Autodesk Inventor part; units mm, degrees
ref_plane "YZ Plane" through (0, 0, 0) normal (1, 0, 0) x (0, 1, 0)
ref_plane "XZ Plane" through (0, 0, 0) normal (0, 1, 0) x (-1, 0, 0)
ref_plane "XY Plane" through (0, 0, 0) normal (0, 0, 1) x (1, 0, 0)
sketch "Sketch1" plane through (0, 0, 0) normal (0, 1, 0) x (-1, 0, 0)
  line L0 (-50.8, 50.8) -> (-50.8, -50.8)
  line L1 (-50.8, -50.8) -> (50.8, -50.8)
  line L2 (50.8, -50.8) -> (50.8, 50.8)
  line L3 (50.8, 50.8) -> (-50.8, 50.8)
  line L4 (-50.8, 50.8) -> (50.8, -50.8) construction
  line L5 (-50.8, -50.8) -> (50.8, 50.8) construction
  line L6 (-47.625, 47.625) -> (-47.625, -47.625)
  line L7 (-47.625, -47.625) -> (47.625, -47.625)
  line L8 (47.625, -47.625) -> (47.625, 47.625)
  line L9 (47.625, 47.625) -> (-47.625, 47.625)
  line L10 (-47.625, 47.625) -> (47.625, -47.625) construction
  line L11 (-47.625, -47.625) -> (47.625, 47.625) construction
  point P0 (0, 0)
  dimension "d0" = 101.6
  dimension "d1" = 3.175
extrude "Extrusion1" add sketch "Sketch1" along normal blind 609.6
properties part number "AlumPost-4x4x36-1_8" material "Aluminum 6061"
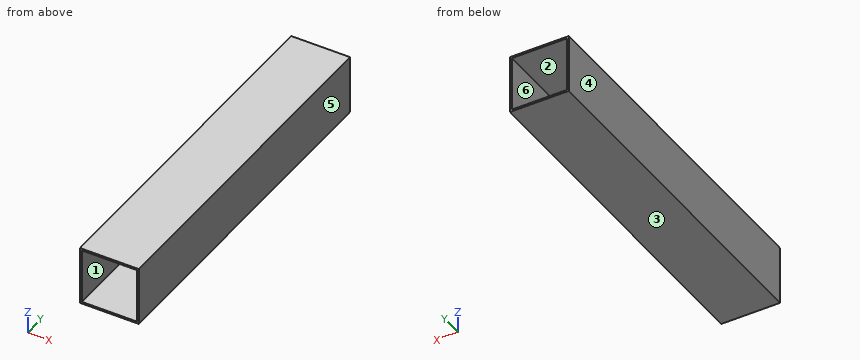
Can you work these out from the model? Positions are in its coordinate system, mm. Face numbers are marked on the shaded views. A direction names the side the tool comes from. Give positions to 0.01 mm unless a question says otherwise; leave off trailing zeros. Order: outer loops, then holes, each group sorted by start corner. A loop starts at its lowest first (then second) coordinate and runs counter-clockwise, first axis right, second up. Notation, with made-up numbers: M 57,25.25 L 79,25.25 A27 cw 79,52.25 Z; hole C 73,84 d9. An arc over 180 degrees is marked long. Use one line per item in the form item = value. Start each with the question number.
Item 1: If we section it at B-B (y = 546): Write out the boundary of the cut face in (x, z) (3 decimals).
Item 2: If we section it at C-C (x = -10): Write out the boundary of the cut face in (y, z) (3 decimals), then the cut area to 3 significant figures.
Item 3: If we section it at A-A (z = 11.5): Write out the boundary of the cut face in (x, y) (3 decimals).
Item 4: If I drill on line 1 along Z through (x, y) = (14.5, 42.5) (3 decimals), over which ranges is the centre line in solid material (lowest first)?
Item 5: For the marked faces 5 and 6, which set-ups out of +Z, -Z, +X, -X, +Y, -Y let a thin tool reach every point of the face, with its end or its side?
Item 6: We'd pull the mould along Z, two halves only. Please class the marked faces 1, 2, 3 and 4: +Z half, -Z half, draft (parallel to the pull), parting line (faces both ways), or undercut.
Outcome:
q1.outline = M -50.8,-50.8 L 50.8,-50.8 L 50.8,50.8 L -50.8,50.8 Z; hole M -47.625,-47.625 L 47.625,-47.625 L 47.625,47.625 L -47.625,47.625 Z
q2.outline = M 0,-50.8 L 609.6,-50.8 L 609.6,-47.625 L 0,-47.625 Z; M 0,47.625 L 609.6,47.625 L 609.6,50.8 L 0,50.8 Z
q2.area = 3,870 mm2
q3.outline = M -50.8,0 L -47.625,0 L -47.625,609.6 L -50.8,609.6 Z; M 47.625,0 L 50.8,0 L 50.8,609.6 L 47.625,609.6 Z
q4.line_1 = -50.8 to -47.625, 47.625 to 50.8
q5.face_5 = +Z, -Z, +X, +Y, -Y
q5.face_6 = +Y, -Y
q6.face_1 = undercut
q6.face_2 = undercut
q6.face_3 = -Z half
q6.face_4 = draft
